For this review, take the finished solid that the model builds, in its own axes (mm). Face numbers are marked on the shaded views. A direction names the side the tool comes from. Coordinates: 2 decimals unless noted, no trailing zeros. Loops run counter-clockwise (first coordinate to the right, second up) from the corner with the lowest first, then second, coordinate; pieces in that order, holes last. Notation, with made-up numbers: (62, 80.5) - (106, 80.5) arc R22 ccw to (106, 114.5) - close; hole circle Ø5 at (77, 19.25). An arc over 180 degrees is marked (long way). Answer as a JSON object with one key per item and string values. Group by question number.
Item 1: Tool access review of the marked faces 1, 2 and 3: name each direction out of +Z, -Z, +X, -X, +Y, -Y from which nothing blocks a thin tool from reaching the whole face with its end or side.
Item 2: To check wall thickness, follow line 1 (X direction, y = 116, z = 11); line 2 (Y direction, x = 102.5, z = 22.5); line 3 (X direction, y = 124, z = 19). State the ranges of each line that lie inside material, in increasing order.
Item 3: We need section B-B (y = 150.5). Give the boundary of the cut face in (x, z), then the cut area to 4 significant figures.
Item 4: We need section C-C (y = 183). Give the boundary of the cut face in (x, z).
Item 5: Clearance check with flat-ended pins moving along their axes: pin 1 (1.2 mm diameter, centred on x = 70.5, z = 0.5, fed in from -Y); pin 2 (6 mm diameter, centred on x = 19.5, z = 17, fed in from -Y); pin 3 (1.6 mm diameter, centred on y = 205, z = 0.5, fed in from +X); pin 4 (13 mm diameter, centred on y = 117.505, z = 25, fed in from -X) (1 decimal). State where each tip first meets the part, or that it passes through.
Item 6: We need section D-D (z = 8). Give the boundary of the cut face in (x, y) (3 decimals), then the cut area to 3 significant figures.
Item 7: We need section A-A (z = 25). Give the boundary of the cut face in (x, y) (3 decimals), then the cut area to 3 significant figures.
Item 8: Mouldability with a two-part tool opening along Y and no side actions: class the marked faces 4, 5 and 6 as released by +Y, released by -Y, zero draft, split by the parting line, or undercut.
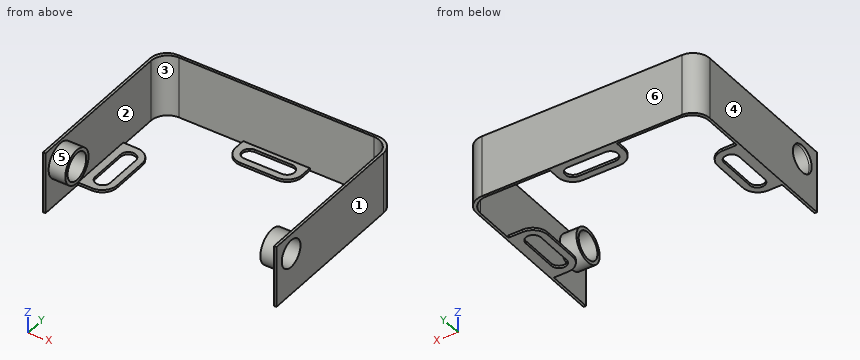
from build123d import *

# Parameters (mm, degrees)
SKIZZE1_W                            = 140
SKIZZE1_H                            = 209.01
SKIZZE1_W_2                          = 137
SKIZZE1_H_2                          = 206.01
AUFSATZ_LINEAR_AUSTRAGEN1_DEPTH      = 37
VERRUNDUNG1_R                        = 10
SCHNITT_LINEAR_AUSTRAGEN2_DEPTH      = 255.27186258
SCHNITT_LINEAR_AUSTRAGEN2_DEPTH_BACK = 255.27186258
SKIZZE4_R                            = 8.25
AUFSATZ_LINEAR_AUSTRAGEN3_DEPTH      = 1.5
SCHNITT_LINEAR_AUSTRAGEN3_DEPTH      = 255.057926662
SCHNITT_LINEAR_AUSTRAGEN3_DEPTH_BACK = 255.057926662
SKIZZE6_W                            = 230.516002865
SKIZZE6_H                            = 119.565202556
AUFSATZ_LINEAR_START                 = 10
SKIZZE8_R                            = 10.25
SKIZZE8_R_2                          = 8.25
AUFSATZ_LINEAR_AUSTRAGEN5_DEPTH      = 10


with BuildPart() as part:
    # Skizze1 → Aufsatz-Linear austragen1 (new body)
    with BuildSketch(Plane.XY):
        with Locations((70, 104.505)):
            Rectangle(SKIZZE1_W, SKIZZE1_H)
        with Locations((70, 104.505)):
            Rectangle(SKIZZE1_W_2, SKIZZE1_H_2, mode=Mode.SUBTRACT)
    extrude(amount=AUFSATZ_LINEAR_AUSTRAGEN1_DEPTH)

    # Verrundung1
    verrundung1_edges = [part.edges().sort_by_distance(p)[0] for p in [
        (1.5, 207.51, 18.5),
        (1.5, 1.5, 18.5),
        (138.5, 1.5, 18.5),
        (138.5, 207.51, 18.5),
        (0, 209.01, 18.5),
        (140, 209.01, 18.5),
        (140, 0, 18.5),
        (0, 0, 18.5),
    ]]
    fillet(verrundung1_edges, radius=VERRUNDUNG1_R)

    # Skizze4 → Schnitt-Linear austragen2 (cut, two sides: drawn at the far end of the back side and taken through both)
    with BuildSketch(Plane(origin=(140, 0, 0), x_dir=(0, 0, -1), z_dir=(1, 0, 0)).offset(-SCHNITT_LINEAR_AUSTRAGEN2_DEPTH_BACK)):
        with Locations(Location((-25, 117.505, 0), (0, 0, 270))):
            Circle(SKIZZE4_R)
        with Locations(Location((-25, 91.505, 0), (0, 0, 270))):
            Circle(SKIZZE4_R)
    extrude(amount=SCHNITT_LINEAR_AUSTRAGEN2_DEPTH + SCHNITT_LINEAR_AUSTRAGEN2_DEPTH_BACK, mode=Mode.SUBTRACT)

    # Skizze5 → Aufsatz-Linear austragen3 (add)
    # profile 1 of 5: a face of its own
    with BuildSketch(Plane(origin=(0, 0, 0), x_dir=(-1, 0, 0), z_dir=(0, 0, -1))):
        with BuildLine():
            Line((-140, 173.01), (-130, 173.01))
            ThreePointArc((-130, 173.01), (-123.636038969, 170.373961031), (-121, 164.01))
            Line((-121, 164.01), (-121, 142.01))
            ThreePointArc((-121, 142.01), (-123.636038969, 135.646038969), (-130, 133.01))
            Line((-130, 133.01), (-140, 133.01))
            Line((-140, 133.01), (-140, 173.01))
        make_face()
        with BuildLine():
            Line((-125, 164.26), (-125, 141.76))
            ThreePointArc((-125, 141.76), (-129.5, 137.26), (-134, 141.76))
            Line((-134, 141.76), (-134, 164.26))
            ThreePointArc((-134, 164.26), (-129.5, 168.76), (-125, 164.26))
        make_face(mode=Mode.SUBTRACT)
    # profile 2 of 5: a face of its own
    with BuildSketch(Plane(origin=(0, 0, 0), x_dir=(-1, 0, 0), z_dir=(0, 0, -1))):
        with BuildLine():
            Line((-90, 209.01), (-90, 200.82))
            ThreePointArc((-90, 200.82), (-87.363961031, 194.456038969), (-81, 191.82))
            Line((-81, 191.82), (-59, 191.82))
            ThreePointArc((-59, 191.82), (-52.636038969, 194.456038969), (-50, 200.82))
            Line((-50, 200.82), (-50, 209.01))
            Line((-50, 209.01), (-90, 209.01))
        make_face()
        with BuildLine():
            Line((-58.75, 204.82), (-81.25, 204.82))
            ThreePointArc((-81.25, 204.82), (-85.75, 200.32), (-81.25, 195.82))
            Line((-81.25, 195.82), (-58.75, 195.82))
            ThreePointArc((-58.75, 195.82), (-54.25, 200.32), (-58.75, 204.82))
        make_face(mode=Mode.SUBTRACT)
    # profile 3 of 5: a face of its own
    with BuildSketch(Plane(origin=(0, 0, 0), x_dir=(-1, 0, 0), z_dir=(0, 0, -1))):
        with BuildLine():
            Line((-19, 164.01), (-19, 142.01))
            ThreePointArc((-19, 142.01), (-16.363961031, 135.646038969), (-10, 133.01))
            Line((-10, 133.01), (0, 133.01))
            Line((0, 133.01), (0, 173.01))
            Line((0, 173.01), (-10, 173.01))
            ThreePointArc((-10, 173.01), (-16.363961031, 170.373961031), (-19, 164.01))
        make_face()
        with BuildLine():
            Line((-15, 164.26), (-15, 141.76))
            ThreePointArc((-15, 141.76), (-10.5, 137.26), (-6, 141.76))
            Line((-6, 141.76), (-6, 164.26))
            ThreePointArc((-6, 164.26), (-10.5, 168.76), (-15, 164.26))
        make_face(mode=Mode.SUBTRACT)
    # profile 4 of 5: a face of its own
    with BuildSketch(Plane(origin=(0, 0, 0), x_dir=(-1, 0, 0), z_dir=(0, 0, -1))):
        with BuildLine():
            Line((0, 36), (-10, 36))
            ThreePointArc((-10, 36), (-16.363961031, 38.636038969), (-19, 45))
            Line((-19, 45), (-19, 67))
            ThreePointArc((-19, 67), (-16.363961031, 73.363961031), (-10, 76))
            Line((-10, 76), (0, 76))
            Line((0, 76), (0, 36))
        make_face()
        with BuildLine():
            Line((-15, 44.75), (-15, 67.25))
            ThreePointArc((-15, 67.25), (-10.5, 71.75), (-6, 67.25))
            Line((-6, 67.25), (-6, 44.75))
            ThreePointArc((-6, 44.75), (-10.5, 40.25), (-15, 44.75))
        make_face(mode=Mode.SUBTRACT)
    # profile 5 of 5: a face of its own
    with BuildSketch(Plane(origin=(0, 0, 0), x_dir=(-1, 0, 0), z_dir=(0, 0, -1))):
        with BuildLine():
            Line((-121, 45), (-121, 67))
            ThreePointArc((-121, 67), (-123.636038969, 73.363961031), (-130, 76))
            Line((-130, 76), (-140, 76))
            Line((-140, 76), (-140, 36))
            Line((-140, 36), (-130, 36))
            ThreePointArc((-130, 36), (-123.636038969, 38.636038969), (-121, 45))
        make_face()
        with BuildLine():
            Line((-125, 44.75), (-125, 67.25))
            ThreePointArc((-125, 67.25), (-129.5, 71.75), (-134, 67.25))
            Line((-134, 67.25), (-134, 44.75))
            ThreePointArc((-134, 44.75), (-129.5, 40.25), (-125, 44.75))
        make_face(mode=Mode.SUBTRACT)
    extrude(amount=-AUFSATZ_LINEAR_AUSTRAGEN3_DEPTH)

    # Skizze6 → Schnitt-Linear austragen3 (cut, two sides: drawn at the far end of the back side and taken through both)
    with BuildSketch(Plane.XY.offset(1.5).offset(-SCHNITT_LINEAR_AUSTRAGEN3_DEPTH_BACK)):
        with Locations((84.29357918, 44.722398722)):
            Rectangle(SKIZZE6_W, SKIZZE6_H)
    extrude(amount=SCHNITT_LINEAR_AUSTRAGEN3_DEPTH + SCHNITT_LINEAR_AUSTRAGEN3_DEPTH_BACK, mode=Mode.SUBTRACT)

    # Skizze8 → Aufsatz-Linear austragen5 (add)
    with BuildSketch(Plane(origin=(1.5, 0, 0), x_dir=(0, 0, -1), z_dir=(1, 0, 0)).offset(AUFSATZ_LINEAR_START)):
        with Locations(Location((-25, 117.505, 0), (0, 0, 90))):
            Circle(SKIZZE8_R)
        with Locations(Location((-25, 117.505, 0), (0, 0, 270))):
            Circle(SKIZZE8_R_2, mode=Mode.SUBTRACT)
    aufsatz_linear_austragen5 = extrude(amount=-AUFSATZ_LINEAR_AUSTRAGEN5_DEPTH)

    # Spiegeln1: Aufsatz-Linear austragen5 across plane
    add(aufsatz_linear_austragen5.mirror(Plane.ZY.offset(-70)))


solid = part.part
Check sheet entries:
{
 "1": {"face 1": "+Z, -Z, +X, +Y, -Y", "face 2": "none", "face 3": "+Z, -Z"},
 "2": {"line 1": "x = 0 to 1.5, 138.5 to 140", "line 2": "y = 207.51 to 209.01", "line 3": "x = 0 to 11.5, 128.5 to 140"},
 "3": {"outline": "(0, 0) - (6, 0) - (6, 1.5) - (1.5, 1.5) - (1.5, 37) - (0, 37) - close; (15, 0) - (19, 0) - (19, 1.5) - (15, 1.5) - close; (121, 0) - (125, 0) - (125, 1.5) - (121, 1.5) - close; (134, 0) - (140, 0) - (140, 37) - (138.5, 37) - (138.5, 1.5) - (134, 1.5) - close", "area": "136.5 mm2"},
 "4": {"outline": "(0, 0) - (1.5, 0) - (1.5, 37) - (0, 37) - close; (138.5, 0) - (140, 0) - (140, 37) - (138.5, 37) - close"},
 "5": {"pin 1": "stops at y = 191.82", "pin 2": "stops at y = 207.51", "pin 3": "stops at x = 138.55", "pin 4": "passes through"},
 "6": {"outline": "(0, 104.505) - (1.5, 104.505) - (1.5, 197.51) arc R10 cw to (11.5, 207.51) - (128.5, 207.51) arc R10 cw to (138.5, 197.51) - (138.5, 104.505) - (140, 104.505) - (140, 199.01) arc R10 ccw to (130, 209.01) - (10, 209.01) arc R10 ccw to (0, 199.01) - close", "area": "519 mm2"},
 "7": {"outline": "(0, 104.505) - (1.5, 104.505) - (1.5, 107.255) - (11.5, 107.255) - (11.5, 109.255) - (0, 109.255) - close; (0, 125.755) - (11.5, 125.755) - (11.5, 127.755) - (1.5, 127.755) - (1.5, 197.51) arc R10 cw to (11.5, 207.51) - (128.5, 207.51) arc R10 cw to (138.5, 197.51) - (138.5, 127.755) - (128.5, 127.755) - (128.5, 125.755) - (140, 125.755) - (140, 199.01) arc R10 ccw to (130, 209.01) - (10, 209.01) arc R10 ccw to (0, 199.01) - close; (128.5, 107.255) - (138.5, 107.255) - (138.5, 104.505) - (140, 104.505) - (140, 109.255) - (128.5, 109.255) - close", "area": "550 mm2"},
 "8": {"face 4": "zero draft", "face 5": "undercut", "face 6": "released by +Y"}
}
